from build123d import *

# Parameters (mm, degrees)
SKETCH1_R                 = 34.544
SKETCH1_W                 = 38.1
SKETCH1_H                 = 25.4
BOSS_EXTRUDE1_DEPTH       = 6.35
BOSS_EXTRUDE1_DEPTH_BACK  = 12.7
CUT_EXTRUDE1_START        = -12.7
SKETCH2_W                 = 38.1
SKETCH2_H                 = 25.4
CUT_EXTRUDE1_DEPTH        = 12.7
SKETCH3_R                 = 39.3065
SKETCH3_R_2               = 34.544
BOSS_EXTRUDE3_DEPTH       = 17.526
SKETCH4_R                 = 34.544
SKETCH4_R_2               = 28.194
BOSS_EXTRUDE4_DEPTH       = 1.5875
BOSS_EXTRUDE10_DEPTH      = 6.35
BOSS_EXTRUDE10_DEPTH_BACK = 2.00152
F_5_16_18_TAPPED_HOLE6_D  = 6.5278
FILLET5_R                 = 2.54
FILLET6_R                 = 2.54
BOSS_EXTRUDE9_DEPTH       = 12.7
BOSS_EXTRUDE9_DEPTH_BACK  = 6.35
FILLET4_R                 = 2.54


with BuildPart() as part:
    # Sketch1 → Boss-Extrude1 (new body, two sides)
    with BuildSketch(Plane.XY) as boss_extrude1_sk:
        with BuildLine():
            Line((-1564.55033403, 132.369836169), (-1537.788605326, 207.210066144))
            ThreePointArc((-1537.788605326, 207.210066144), (-1535.565917531, 218.059885236), (-1536.458056316, 229.099042982))
            Line((-1536.458056316, 229.099042982), (-1549.023662845, 284.769836169))
            Line((-1549.023662845, 284.769836169), (-1587.123662845, 284.769836169))
            Line((-1587.123662845, 284.769836169), (-1610.117979725, 237.697060793))
            ThreePointArc((-1610.117979725, 237.697060793), (-1613.600930979, 226.72878162), (-1613.757951397, 215.221851446))
            Line((-1613.757951397, 215.221851446), (-1602.65033403, 132.369836169))
            Line((-1602.65033403, 132.369836169), (-1564.55033403, 132.369836169))
        make_face()
        with Locations((-1574.8, 220.444778325)):
            Circle(SKETCH1_R, mode=Mode.SUBTRACT)
        with BuildLine():
            Line((-1565.649571077, 143.440187232), (-1574.961325855, 181.138609391))
            ThreePointArc((-1574.961325855, 181.138609391), (-1560.844896551, 183.698948221), (-1548.587601226, 191.154658954))
            Line((-1548.587601226, 191.154658954), (-1565.649571077, 143.440187232))
        make_face(mode=Mode.SUBTRACT)
        with BuildLine():
            Line((-1599.316994088, 143.347801615), (-1606.545707049, 197.266965093))
            ThreePointArc((-1606.545707049, 197.266965093), (-1595.557832884, 187.066442294), (-1581.549876664, 181.722173721))
            Line((-1581.549876664, 181.722173721), (-1599.316994088, 143.347801615))
        make_face(mode=Mode.SUBTRACT)
        Polygon((-1582.899237332, 280.007336169), (-1554.644379273, 280.007336169), (-1571.531413288, 257.824658876), align=None, mode=Mode.SUBTRACT)
        Polygon((-1567.361913884, 137.132336169), (-1578.262893423, 181.264697727), (-1598.695927423, 137.132336169), align=None, mode=Mode.SUBTRACT)
        with BuildLine():
            Line((-1545.232831462, 246.344266484), (-1552.333167166, 277.801667254))
            Line((-1552.333167166, 277.801667254), (-1566.714355054, 258.910650056))
            ThreePointArc((-1566.714355054, 258.910650056), (-1554.952781307, 254.372478695), (-1545.232831462, 246.344266484))
        make_face(mode=Mode.SUBTRACT)
        with BuildLine():
            Line((-1576.07575514, 259.730569536), (-1585.280544841, 277.692395712))
            Line((-1585.280544841, 277.692395712), (-1597.607290416, 252.457720179))
            ThreePointArc((-1597.607290416, 252.457720179), (-1587.378626922, 257.684261229), (-1576.07575514, 259.730569536))
        make_face(mode=Mode.SUBTRACT)
        with Locations((-1568.073662845, 297.469836169)):
            Rectangle(SKETCH1_W, SKETCH1_H)
        with Locations((-1583.60033403, 119.669836169)):
            Rectangle(SKETCH1_W, SKETCH1_H)
    extrude(amount=BOSS_EXTRUDE1_DEPTH)
    extrude(boss_extrude1_sk.sketch, amount=-BOSS_EXTRUDE1_DEPTH_BACK)

    # Sketch2 → Cut-Extrude1 (cut)
    with BuildSketch(Plane(origin=(0, 0, -12.7), x_dir=(-1, 0, 0), z_dir=(0, 0, -1)).offset(CUT_EXTRUDE1_START)):
        with Locations((1568.073662845, 297.469836169)):
            Rectangle(SKETCH2_W, SKETCH2_H)
        with Locations((1583.60033403, 119.669836169)):
            Rectangle(SKETCH2_W, SKETCH2_H)
    extrude(amount=CUT_EXTRUDE1_DEPTH, mode=Mode.SUBTRACT)

    # Sketch3 → Boss-Extrude3 (add)
    with BuildSketch(Plane(origin=(0, 0, -12.7), x_dir=(-1, 0, 0), z_dir=(0, 0, -1))):
        with Locations((1574.8, 220.444778325)):
            Circle(SKETCH3_R)
        with Locations((1574.8, 220.444778325)):
            Circle(SKETCH3_R_2, mode=Mode.SUBTRACT)
    extrude(amount=BOSS_EXTRUDE3_DEPTH)

    # Sketch4 → Boss-Extrude4 (add, symmetric)
    with BuildSketch(Plane(origin=(0, 0, -11.938), x_dir=(-1, 0, 0), z_dir=(0, 0, -1))):
        with Locations((1574.8, 220.444778325)):
            Circle(SKETCH4_R)
        with Locations((1574.8, 220.444778325)):
            Circle(SKETCH4_R_2, mode=Mode.SUBTRACT)
    extrude(amount=BOSS_EXTRUDE4_DEPTH, both=True)

    # Sketch50 → Boss-Extrude10 (add, two sides)
    with BuildSketch(Plane.XY) as boss_extrude10_sk:
        with BuildLine():
            Line((-1541.32707152, 250.670778325), (-1536.458056316, 229.099042982))
            ThreePointArc((-1536.458056316, 229.099042982), (-1535.565917531, 218.059885236), (-1537.788605326, 207.210066144))
            Line((-1537.788605326, 207.210066144), (-1543.86443159, 190.218778325))
            Line((-1543.86443159, 190.218778325), (-1546.702760944, 182.281278325))
            Line((-1546.702760944, 182.281278325), (-1499.66049752, 182.281278325))
            ThreePointArc((-1499.66049752, 182.281278325), (-1491.723009436, 190.232532365), (-1499.688005558, 198.156230659))
            ThreePointArc((-1499.688005558, 198.156230659), (-1512.984254944, 220.398966531), (-1499.842491961, 242.733325991))
            ThreePointArc((-1499.842491961, 242.733325991), (-1491.932511916, 250.684532365), (-1499.87, 258.608278325))
            Line((-1499.87, 258.608278325), (-1543.118666289, 258.608278325))
            Line((-1543.118666289, 258.608278325), (-1541.32707152, 250.670778325))
        make_face()
        with BuildLine():
            Line((-1535.178710458, 252.258278325), (-1507.647129933, 252.258278325))
            ThreePointArc((-1507.647129933, 252.258278325), (-1507.638572597, 249.041917968), (-1506.354439589, 246.09301146))
            ThreePointArc((-1506.354439589, 246.09301146), (-1513.671222734, 238.58285904), (-1518.142792697, 229.099042982))
            ThreePointArc((-1518.142792697, 229.099042982), (-1524.047084498, 224.378892556), (-1529.9513763, 229.099042982))
            Line((-1529.9513763, 229.099042982), (-1535.178710458, 252.258278325))
        make_face(mode=Mode.SUBTRACT)
        with BuildLine():
            Line((-1507.647129933, 188.631278325), (-1537.68832903, 188.631278325))
            Line((-1537.68832903, 188.631278325), (-1531.044836894, 207.210066144))
            ThreePointArc((-1531.044836894, 207.210066144), (-1523.771769284, 212.333403895), (-1516.498701674, 207.210066144))
            ThreePointArc((-1516.498701674, 207.210066144), (-1512.22122179, 200.353921044), (-1506.354439589, 194.79654519))
            ThreePointArc((-1506.354439589, 194.79654519), (-1507.638572597, 191.847638682), (-1507.647129933, 188.631278325))
        make_face(mode=Mode.SUBTRACT)
    extrude(amount=BOSS_EXTRUDE10_DEPTH)
    extrude(boss_extrude10_sk.sketch, amount=-BOSS_EXTRUDE10_DEPTH_BACK)

    # 5/16-18 Tapped Hole6 (through all)
    with Locations(Plane.XY.offset(6.35)):
        with Locations((-1499.87, 250.670778325), (-1499.66049752, 190.218778325)):
            Hole(F_5_16_18_TAPPED_HOLE6_D / 2)

    # Fillet5
    fillet5_edges = [part.edges().sort_by_distance(p)[0] for p in [
        (-1506.354439589, 246.09301146, 2.17424),
        (-1507.647129933, 252.258278325, 2.17424),
        (-1506.354439589, 194.79654519, 2.17424),
        (-1507.647129933, 188.631278325, 2.17424),
    ]]
    fillet(fillet5_edges, radius=FILLET5_R)

    # Fillet6
    fillet6_edges = [part.edges().sort_by_distance(p)[0] for p in [
        (-1535.178710458, 252.258278325, 2.17424),
        (-1537.68832903, 188.631278325, 2.17424),
    ]]
    fillet(fillet6_edges, radius=FILLET6_R)

    # rod connection → Boss-Extrude9 (add, two sides)
    with BuildSketch(Plane(origin=(0, 0, 0), x_dir=(-1, 0, 0), z_dir=(0, 0, -1))) as boss_extrude9_sk:
        Polygon((1647.10033403, 161.645888869), (1606.575249921, 161.645888869), (1607.213738044, 166.408388869), (1658.013738044, 166.408388869), (1658.013738044, 161.645888869), align=None)
        Polygon((1647.10033403, 152.120888869), (1605.298273676, 152.120888869), (1604.659785553, 147.358388869), (1658.013738044, 147.358388869), (1658.013738044, 152.120888869), align=None)
    extrude(amount=BOSS_EXTRUDE9_DEPTH)
    extrude(boss_extrude9_sk.sketch, amount=-BOSS_EXTRUDE9_DEPTH_BACK)

    # Fillet4
    fillet4_edges = [part.edges().sort_by_distance(p)[0] for p in [
        (-1605.298273676, 152.120888869, -3.175),
        (-1604.659785553, 147.358388869, -3.175),
        (-1607.213738044, 166.408388869, -3.175),
        (-1606.575249921, 161.645888869, -3.175),
    ]]
    fillet(fillet4_edges, radius=FILLET4_R)


solid = part.part
Geometry check sheet. Reference: the model listing, model coordinates, mm. A direction names the side the tool comes from. Round coordinates to 2 decimals unless told otherwise and drop trailing zeros. Loops run counter-clockwise (first coordinate to the right, second up) from the corner with the lowest first, then second, coordinate; pieces in that order, holes last.
Item 1: Access from +Z, -Z, +X, -X, +Y, -Y to the whole of each face (thin tool, end or side, straight path). Record for faces 5 (the flat face through (-1583, 132.37, -6)), 6 (the flat face through (-1546, 221, -13.526)), 7 (the flat face through (-1632, 147.358, -3)), 8 (the flat face through (-1522, 188.631, 2)).
Item 2: Cross-section at B-B on x = -1559. Count the separate pieces of the cut face and the enclosed holes in it, then the cut area to 3 significant figures.
Item 3: Gauge pin test, flat ends, axial feed: pin 1 (21 mm diameter, centred on x = -1625.5, z = -3, fed in from -Y); pin 2 (5 mm diameter, centred on y = 275.5, z = -12, fed in from -X); pin 3 (9.5 mm diameter, centred on x = -1581, z = -1.5, fed in from +Y); pin 4 (4 mm diameter, centred on x = -1518.5, z = 3.5, fed in from -Y). Record the tip position at first contact, or that the pin passes through.
Item 4: Thickness scan on line 1 (Y direction, x = -1574, z = -25); line 2 (Y direction, x = -1585.5, z = -5); line 3 (X direction, y = 267, z = 0). Record the ranges inside material, lowest first.
Item 5: Cross-section at D-D on z = -22. Record the boundary of the cut face in (x, y).
Item 6: Cross-section at C-C on y = 129.5. Record the boundary of the cut face in (x, z).
Item 7: Cross-section at A-A on x = -1522. Record the boundary of the cut face in (y, z).
Item 8: Mould release check, pull along Y, two halves, no side actions. Record for faces 1 (the flat face through (-1548.733, 261.853, -3.042)), 2 (the flat face through (-1568, 310.17, 3)), 3 (the flat face through (-1658.014, 164, -3)), 4 (the flat face through (-1572.736, 158.89, -3.042)): pulls with the +Y half, pulls with the -Y half, needs draft (parallel to the pull), parting line crosses it, or undercut.
Answer sheet:
1. face 5: -Z, +X, -X, -Y
1. face 6: -Z
1. face 7: +Z, -Z, -X, -Y
1. face 8: +Z, -Z
2. separate pieces: 5
2. enclosed holes: 0
2. area: 1,050 mm2
3. pin 1: stops at y = 147.36
3. pin 2: stops at x = -1592.87
3. pin 3: stops at y = 310.17
3. pin 4: stops at y = 182.28
4. line 1: y = 181.15 to 185.91, 254.98 to 259.74
4. line 2: y = 132.37 to 137.13, 165.63 to 173.19, 182.62 to 187.6, 253.29 to 258.27, 277.24 to 284.77
4. line 3: x = -1595.8 to -1590.5, -1579.8 to -1576.23, -1564.55 to -1560.56, -1549.9 to -1545.01
5. outline: circle Ø78.61 at (-1574.8, 220.44); hole circle Ø69.09 at (-1574.8, 220.44)
6. outline: (-1602.65, 0) - (-1564.55, 0) - (-1564.55, 6.35) - (-1602.65, 6.35) - close
7. outline: (182.28, -2) - (188.63, -2) - (188.63, 6.35) - (182.28, 6.35) - close; (212.13, -2) - (224.74, -2) - (224.74, 6.35) - (212.13, 6.35) - close; (252.26, -2) - (258.61, -2) - (258.61, 6.35) - (252.26, 6.35) - close
8. face 1: undercut
8. face 2: pulls with the +Y half
8. face 3: needs draft
8. face 4: undercut
